Autodesk Inventor part; units mm, degrees
ref_plane "YZ Plane" through (0, 0, 0) normal (1, 0, 0) x (0, 1, 0)
ref_plane "XZ Plane" through (0, 0, 0) normal (0, 1, 0) x (-1, 0, 0)
ref_plane "XY Plane" through (0, 0, 0) normal (0, 0, 1) x (1, 0, 0)
sketch "Náčrt1" plane through (0, 0, 0) normal (0, 0, 1) x (1, 0, 0)
  line L0 (-6.325, 3.375) -> (6.325, 3.375)
  line L1 (6.325, 3.375) -> (6.325, -3.375)
  line L2 (6.325, -3.375) -> (-6.325, -3.375)
  line L3 (-6.325, -3.375) -> (-6.325, 3.375)
  line L4 (0, 0) -> (-6.325, 3.375) construction
  line L5 (6.325, 3.375) -> (0, 0) construction
  line L6 (6.325, -3.375) -> (0, 0) construction
  dimension "d0" = 12.65
  dimension "d1" = 6.75
extrude "Vysunutí1" add sketch "Náčrt1" along normal blind 6.4
sketch "Náčrt2" plane through (0, 0, 6.4) normal (0, 0, 1) x (1, 0, 0)
  line L0 (-9.75, 3.375) -> (9.75, 3.375)
  line L1 (9.75, 3.375) -> (9.75, -3.375)
  line L2 (9.75, -3.375) -> (-9.75, -3.375)
  line L3 (-9.75, -3.375) -> (-9.75, 3.375)
  line L4 (6.325, -3.375) -> (6.325, 3.375)
  line L5 (6.325, 0) -> (9.75, 0) construction
  line L6 (-9.75, 0) -> (-6.325, 0) construction
  line L7 (-6.325, 3.375) -> (-6.325, -3.375)
  point P0 (0, 0)
  dimension "d4" = 19.5
extrude "Vysunutí2" add sketch "Náčrt2" along normal blind 0.3
sketch "Náčrt3" plane through (0, 0, 6.7) normal (0, 0, 1) x (1, 0, 0)
  circle A0 centre (-7.65, 0) radius 1.325
  circle A1 centre (7.65, 0) radius 1.325
  line L0 (-6.325, 3.375) -> (-6.325, -3.375)
  line L1 (6.325, -3.375) -> (6.325, 3.375)
  line L2 (-7.65, 1.325) -> (-9.75, 1.325)
  line L3 (-9.75, 3.375) -> (-9.75, -3.375)
  line L4 (-7.65, -1.325) -> (-9.75, -1.325)
  line L5 (7.65, 1.325) -> (9.75, 1.325)
  line L6 (9.75, -3.375) -> (9.75, 3.375)
  line L7 (7.65, -1.325) -> (9.75, -1.325)
  point P0 (0, 0)
  dimension "d7" = 2.65
extrude "Vysunutí3" cut sketch "Náčrt3" against normal up to surface (0.3 mm away)
sketch "Náčrt4" plane through (-6.325, -3.375, 0) normal (-1, 0, 0) x (0, 0, 1)
  line L0 (0, 0) -> (0, 6.75)
  line L1 (-1.5, 4.375) -> (-4.2, 4.375)
  line L2 (-4.2, 4.375) -> (-4.2, 2.375)
  line L3 (-4.2, 2.375) -> (-1.5, 2.375)
  line L4 (-3.45, 2.875) -> (-1.75, 2.875)
  line L5 (-1.75, 2.875) -> (-1.75, 3.875)
  line L6 (-1.75, 3.875) -> (-3.45, 3.875)
  line L7 (-3.45, 3.875) -> (-3.45, 2.875)
  line L8 (0, 0) -> (6.4, 0)
  line L9 (-4.2, 2.375) -> (0, 0) construction
  line L10 (-4.2, 4.375) -> (0, 6.75) construction
  line L11 (-1.5, 4.375) -> (-1, 4.525)
  line L12 (-1.5, 2.375) -> (-1, 2.225)
  line L13 (-1, 4.525) -> (-0.1, 4.525)
  line L14 (-0.1, 4.525) -> (-0.7641, 5.0796)
  arc A0 (-0.6648, 5.25) -> (-0.7641, 5.0796) centre (-0.7, 5.1564) ccw
  line L15 (-0.6648, 5.25) -> (0, 5)
  line L16 (-1, 2.225) -> (-0.1, 2.225)
  line L17 (-0.1, 2.225) -> (-0.7641, 1.6704)
  arc A1 (-0.7641, 1.6704) -> (-0.6648, 1.5) centre (-0.7, 1.5936) ccw
  line L18 (-0.6648, 1.5) -> (0, 1.75)
  line L19 (-0.1, 4.525) -> (0, 5) construction
  line L20 (-0.1, 2.225) -> (0, 1.75) construction
  point P0 (0, 3.375)
  dimension "d10" = 2
  dimension "d11" = 4.2
  dimension "d12" = 0.5
  dimension "d13" = 0.5
  dimension "d14" = 1.75
  dimension "d16" = 0.75
  dimension "d18" = 1.5
  dimension "d19" = 2.3
  dimension "d20" = 1
  dimension "d22" = 0.8
  dimension "d23" = 3.75
  dimension "d24" = 0.1
  dimension "d25" = 3.25
  dimension "d27" = 0.1
extrude "Vysunutí4" add sketch "Náčrt4" against normal up to surface (12.65 mm away)
sketch "Náčrt5" plane through (-6.325, -3.375, 0) normal (0, -1, 0) x (1, 0, 0)
  line L0 (12.65, 0) -> (12.65, 6.4)
  line L1 (12.65, 0) -> (11.525, 0)
  line L2 (11.525, 0) -> (11.525, -4.2)
  line L3 (11.525, -4.2) -> (12.65, -4.2)
  line L4 (12.65, -4.2) -> (12.65, 0)
  line L5 (0, 0) -> (12.65, 0)
  line L6 (10.725, -4.2) -> (6.725, -4.2)
  line L7 (6.725, -4.2) -> (6.725, 0)
  line L8 (6.725, 0) -> (10.725, 0)
  line L9 (10.725, 0) -> (10.725, -4.2)
  line L10 (5.925, -4.2) -> (1.925, -4.2)
  line L11 (1.925, -4.2) -> (1.925, 0)
  line L12 (1.925, 0) -> (5.925, 0)
  line L13 (5.925, 0) -> (5.925, -4.2)
  line L14 (1.125, -4.2) -> (0, -4.2)
  line L15 (0, -4.2) -> (0, 0)
  line L16 (0, 0) -> (1.125, 0)
  line L17 (1.125, 0) -> (1.125, -4.2)
  line L18 (0, -4.2) -> (12.65, -4.2)
  line L19 (11.525, -2.1) -> (10.725, -2.1) construction
  line L20 (6.725, -2.1) -> (5.925, -2.1) construction
  line L21 (1.925, -2.1) -> (1.125, -2.1) construction
  point P0 (6.325, 0)
  point P1 (1.125, 0)
  dimension "d30" = 0.8
  dimension "d31" = 4
extrude "Vysunutí5" cut sketch "Náčrt5" against normal through all contours L4 L3 L2 L1 | L9 L6 L7 L5 | L13 L10 L11 L5 | L17 L14 L15 L5
sketch "Náčrt6" plane through (0, 0, 6.7) normal (0, 0, 1) x (1, 0, 0)
  line L0 (0.85, 1.9) -> (-2.95, 1.9)
  line L1 (-2.95, 1.9) -> (-2.95, -1.9)
  line L2 (-2.95, -1.9) -> (0.85, -1.9)
  line L3 (0.85, -1.9) -> (0.85, 1.9)
  line L4 (-9.75, -1.325) -> (-9.75, -3.375)
  point P0 (0, 0)
  point P1 (0.85, 0)
  dimension "d34" = 3.8
  dimension "d35" = 6.8
extrude "Vysunutí6" add sketch "Náčrt6" along normal blind 5
properties part number "switch"
Geometry: final body of the model. Coordinates: model frame, mm. A direction names the side the tool comes from. Give positions to 0.01 mm unless a question says otherwise; leave off trailing zeros. Loops run counter-clockwise (first coordinate to the right, second up) from the corner with the lowest first, then second, coordinate; pieces in that order, holes last. Notation, with made-up numbers: M 73,62.25 L 110,62.25 A16 cw 110,83.25 Z; hole C 23,39 d1. An arc over 180 degrees is marked long. Put each result on its own line as item: value. Start each with the question number.
1) Pull-direction query (Z, two-part tool) for faces 6 (the flat face through (0, -0.5, -3)), 7 (the flat face through (-8, -2, 6.4)), 8 (the flat face through (-6.325, 0, 3)); classes: pulls with the +Z half, pulls with the -Z half, needs draft (parallel to the pull), parting line crosses it, or undercut.
2) Cut plane C-C (x = -5.5). Output: boundary loops of the cut face in (y, z) (3 decimals), then the cut area to 3 significant figures.
3) Cut plane A-A (y = 2.25). Output: boundary loops of the cut face in (x, z) (3 decimals), then the cut area to 3 significant figures.
4) Contact query for flat-ended pins moving along their axis: pin 1 (1.5 mm diameter, centred on y = 0.5, z = 0, fed in from +X) (3 decimals); pin 2 (0.9 mm diameter, centred on x = -5, z = -2.5, fed in from -Y); pin 3 (0.6 mm diameter, centred on x = -4.5, z = -0.5, fed in from +Y); pin 4 (3.5 mm diameter, centred on x = -4.5, y = 0, fed in from +Z). Output: stop coordinate, or through.
5) Ray query, line 1 along Z through (x, y) = (-5, 0); line 2 along Z through (x, y) = (-3, -1.75); line 3 along Y through (x, z) = (-1.75, 9). Return the intervals inside material, ascending.
6) Access query for faces 1 (the flat face through (0, 0, -1.75)), 2 (the flat face through (-1, -1.9, 9)), 3 (the flat face through (-2.95, 0, 9)), 4 (the flat face through (-8, 2, 6.4)), 5 (the flat face through (5.2, 0, -1)). Directions: +Z, -Z, +X, -X, +Y, -Y. A direction counts if a zero-diameter tool reaches every point of the face in a straight line with its end or side. Return the directions, or none.
7) Cut plane B-B (z = 10.5). Output: boundary loops of the cut face in (x, y).
Verdict:
1. face 6: undercut
1. face 7: pulls with the -Z half
1. face 8: needs draft
2. outline: M -3.375,0 L 3.375,0 L 3.375,6.7 L -3.375,6.7 Z
2. area: 45.2 mm2
3. outline: M -9.75,6.4 L -6.325,6.4 L -6.325,0 L 6.325,0 L 6.325,6.4 L 9.75,6.4 L 9.75,6.7 L -9.75,6.7 Z
3. area: 86.8 mm2
4. pin 1: x = 6.325
4. pin 2: y = -1
4. pin 3: y = 1.88
4. pin 4: z = 11.7
5. line 1: -4.2 to -3.45, -1.75 to 6.7
5. line 2: 0 to 6.7
5. line 3: -1.9 to 1.9
6. face 1: +X, -X
6. face 2: +Z, +X, -X, -Y
6. face 3: +Z, -X, +Y, -Y
6. face 4: -Z, -X, +Y, -Y
6. face 5: -Z, +X, +Y, -Y
7. outline: M -2.95,-1.9 L 0.85,-1.9 L 0.85,1.9 L -2.95,1.9 Z
